For this review, take the finished solid that the model builds, in its own axes (mm). A direction names the side the tool comes from. Round coordinates to 2 decimals unless told otherwise and drop trailing zeros. Loops run counter-clockwise (first coordinate to the right, second up) from the corner with the lowest first, then second, coordinate; pieces in that order, holes last.
1. To check wall thickness, follow line 1 along X through (y, z) = (13, 1.75); line 2 along Y through (x, z) = (71.2, 10.2); line 3 along X through (y, z) = (36.5, 10.25). State the ranges of each line that lie inside material, in increasing order.
2. Clearance check with flat-ended pins moving along their axes: pin 1 Ø3.5 at (x, y) = (-20, 36.7) entering from +Z; pin 2 Ø5 at (x, y) = (71.2, -50.15) entering from +Z; pin 3 Ø3 at (x, y) = (-23, -43) entering from -Z. State where each tip first meets the part, or that it passes through.
3. Consider section A-A on z = 2.75. State how many separate pieces and enclosed holes the cut face has, then the cut area to 3 significant figures.
4. Tool access review of faces 1 (the cylindrical face through (-42.952, 24.051, 4.289)), 2 (the flat face through (22.2, 10.5, 7.7)), 3 (the cylindrical face through (24.148, -41.231, 2.379)): name each direction out of +Z, -Z, +X, -X, +Y, -Y from which nothing blocks a thin tool from reaching the whole face with its end or side.
5. Consider section B-B on y = 36.7. State the section outline as (x, z) points.
from build123d import *

# Parameters (mm, degrees)
SKETCH1_W                                       = 152.4
SKETCH1_H                                       = 114.3
BOSS_EXTRUDE1_DEPTH                             = 12.7
CBORE_FOR_10_SOCKET_HEAD_CAP_SCREW1_D           = 5.1054
CBORE_FOR_10_SOCKET_HEAD_CAP_SCREW1_CBORE_D     = 9.525
CBORE_FOR_10_SOCKET_HEAD_CAP_SCREW1_CBORE_DEPTH = 4.826
CBORE_FOR_M4_SHCS1_D                            = 4.5
CBORE_FOR_M4_SHCS1_CBORE_D                      = 8
CBORE_FOR_M4_SHCS1_CBORE_DEPTH                  = 4
MIRROR2_COPY_1_D                                = 4.5
MIRROR2_COPY_1_CBORE_D                          = 8
MIRROR2_COPY_1_CBORE_DEPTH                      = 4
CBORE_FOR_M5_SHCS1_D                            = 5.5
CBORE_FOR_M5_SHCS1_CBORE_D                      = 10
CBORE_FOR_M5_SHCS1_CBORE_DEPTH                  = 5


with BuildPart() as part:
    # Sketch1 → Boss-Extrude1 (new body)
    with BuildSketch(Plane.XY):
        Rectangle(SKETCH1_W, SKETCH1_H)
    extrude(amount=BOSS_EXTRUDE1_DEPTH)

    # CBORE for #10 Socket Head Cap Screw1 (through all)
    with Locations(Plane(origin=(0, 0, 0), x_dir=(-1, 0, 0), z_dir=(0, 0, -1))):
        with Locations((-20.6375, -6.35), (20.6375, -6.35), (20.6375, -44.45), (-20.6375, -44.45)):
            CounterBoreHole(CBORE_FOR_10_SOCKET_HEAD_CAP_SCREW1_D / 2, CBORE_FOR_10_SOCKET_HEAD_CAP_SCREW1_CBORE_D / 2, CBORE_FOR_10_SOCKET_HEAD_CAP_SCREW1_CBORE_DEPTH)

    # CBORE for M4 SHCS1 (through all)
    with Locations(Plane.XY.offset(12.7)):
        with Locations((-71.2, -50.15), (-45.2, -50.15), (-45.2, -24.15), (-71.2, -24.15)):
            cbore_for_m4_shcs1 = CounterBoreHole(CBORE_FOR_M4_SHCS1_D / 2, CBORE_FOR_M4_SHCS1_CBORE_D / 2, CBORE_FOR_M4_SHCS1_CBORE_DEPTH)

    # Mirror1: CBORE for M4 SHCS1 across plane
    add(cbore_for_m4_shcs1.mirror(Plane.ZX), mode=Mode.SUBTRACT)

    # Mirror2: CBORE for M4 SHCS1 across plane
    add(cbore_for_m4_shcs1.mirror(Plane(origin=(0, 0, 0), x_dir=(0, 0, 1), z_dir=(1, 0, 0))), mode=Mode.SUBTRACT)

    # Mirror2 copy 1 (through all)
    with Locations(Plane(origin=(0, 0, 12.7), x_dir=(-1, 0, 0), z_dir=(0, 0, 1))):
        with Locations((-71.2, -50.15), (-45.2, -50.15), (-45.2, -24.15), (-71.2, -24.15)):
            CounterBoreHole(MIRROR2_COPY_1_D / 2, MIRROR2_COPY_1_CBORE_D / 2, MIRROR2_COPY_1_CBORE_DEPTH)

    # CBORE for M5 SHCS1 (through all)
    with Locations(Plane.XY.offset(12.7)):
        with Locations((-20, 36.7), (20, 36.7), (20, 12.7), (-20, 12.7)):
            CounterBoreHole(CBORE_FOR_M5_SHCS1_D / 2, CBORE_FOR_M5_SHCS1_CBORE_D / 2, CBORE_FOR_M5_SHCS1_CBORE_DEPTH)


solid = part.part
Resolved:
1. line 1: x = -76.2 to -22.73, -17.27 to 17.27, 22.73 to 76.2
1. line 2: y = -57.15 to -54.15, -46.15 to -28.15, -20.15 to 20.15, 28.15 to 46.15, 54.15 to 57.15
1. line 3: x = -76.2 to -25, -15 to 15, 25 to 76.2
2. pin 1: passes through
2. pin 2: stops at z = 8.7
2. pin 3: stops at z = 4.83
3. separate pieces: 1
3. enclosed holes: 24
3. area: 16,800 mm2
4. face 1: +Z, -Z
4. face 2: +Z
4. face 3: -Z
5. outline: (-76.2, 0) - (-22.75, 0) - (-22.75, 7.7) - (-25, 7.7) - (-25, 12.7) - (-76.2, 12.7) - close; (-17.25, 0) - (17.25, 0) - (17.25, 7.7) - (15, 7.7) - (15, 12.7) - (-15, 12.7) - (-15, 7.7) - (-17.25, 7.7) - close; (22.75, 0) - (76.2, 0) - (76.2, 12.7) - (25, 12.7) - (25, 7.7) - (22.75, 7.7) - close
